Geometry check sheet. Reference: drawing and pictorial views, mm from the part's lowest x, y, z. A direction names the side the tool comes from. Round coordinates to 2 decimals unless told otherwise and drop trailing zeros. Order: outer loops, then holes, each group sorted by start corner. A loop starts at its lowest first (then second) coordinate and runs counter-clockwise, first axis right, second up. Notation, with made-up numbers: (86.5, 24) -> (133.5, 24) arc R16 ccw to (133.5, 41) -> close; hole circle Ø7 at (76, -5). An arc over 180 degrees is marked (long way). Put each result on its own line as item: value.
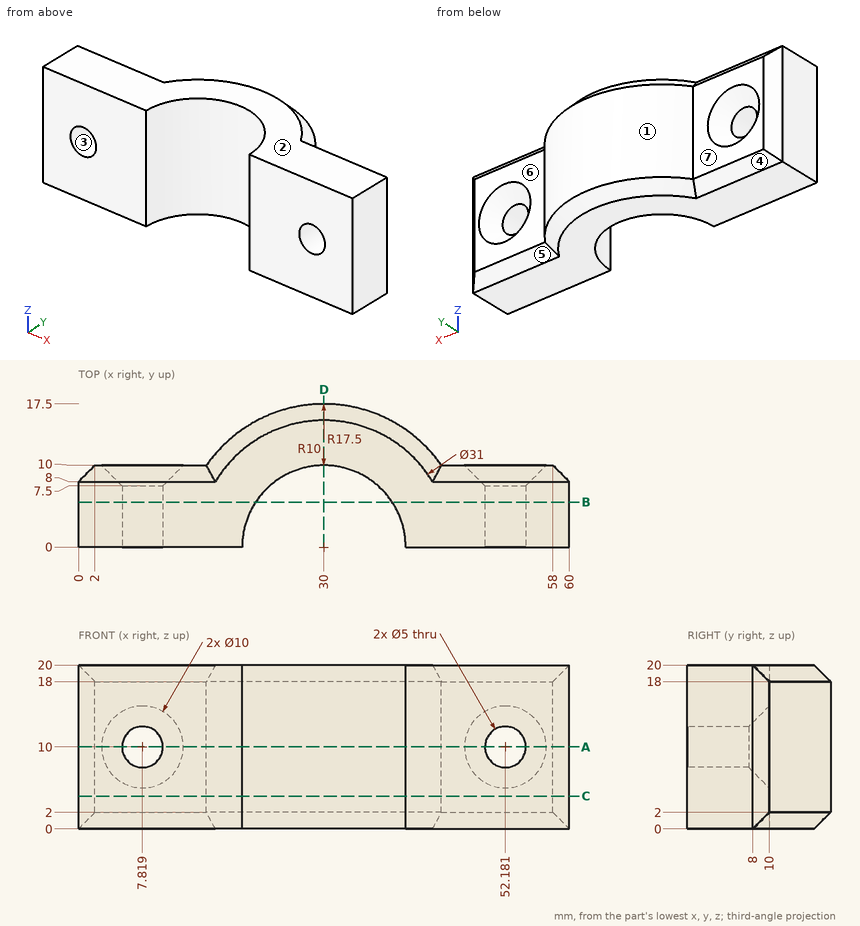
Item 1: Sectioned sample at A-A, the plane z = 10. Record the boundary of the cut face in (x, y).
Geometry check:
outline: (0, 0) -> (5.32, 0) -> (5.32, 7.5) -> (2.82, 10) -> (2, 10) -> (0, 8) -> close; (10.32, 0) -> (20, 0) arc R10 cw to (40, 0) -> (49.68, 0) -> (49.68, 7.5) -> (47.18, 10) -> (44.36, 10) arc R17.5 ccw to (15.64, 10) -> (12.82, 10) -> (10.32, 7.5) -> close; (54.68, 0) -> (60, 0) -> (60, 8) -> (58, 10) -> (57.18, 10) -> (54.68, 7.5) -> close
Item 2: Sectioned sample at B-B, the plane y = 5.5. Record the boundary of the cut face in (x, z), then the cut area to 3 significant figures.
Geometry check:
outline: (0, 0) -> (21.65, 0) -> (21.65, 20) -> (0, 20) -> close; (38.35, 0) -> (60, 0) -> (60, 20) -> (38.35, 20) -> close; hole circle Ø5 at (7.82, 10); hole circle Ø5 at (52.18, 10)
area: 827 mm2
Item 3: Release check for a two-part mould opening along X. For the marked faces 1, 2 and 3 record: pulls with the +X half, pulls with the -X half, needs draft (parallel to the pull), parting line crosses it, or undercut.
Geometry check:
face 1: parting line crosses it
face 2: needs draft
face 3: undercut
Item 4: Sectioned sample at D-D, the plane x = 30. Record the boundary of the cut face in (y, z).
Geometry check:
outline: (10, 0) -> (15.5, 0) -> (17.5, 2) -> (17.5, 18) -> (15.5, 20) -> (10, 20) -> close
Item 5: Material ranges on line 1 along X through (y, z) = (5, 10); line 2 along X through (y, z) = (5.5, 10); line 3 along X through (y, z) = (3.75, 18.5), recorded low to high.
Geometry check:
line 1: 0 to 5.32, 10.32 to 21.34, 38.66 to 49.68, 54.68 to 60
line 2: 0 to 5.32, 10.32 to 21.65, 38.35 to 49.68, 54.68 to 60
line 3: 0 to 20.73, 39.27 to 60
Item 6: Depth check by flat-ended pin: pin 1 Ø11 at (x, z) = (6.5, 6) entering from +Y; pin 2 Ø10 at (x, y) = (9.5, 10) entering from -Z; pin 3 Ø8 at (x, z) = (52.18, 10) entering from +Y. Enter the tip coordinate at first touch or a pass-through.
Geometry check:
pin 1: y = 10
pin 2: z = 0
pin 3: y = 9
Item 7: Sectioned sample at C-C, the plane z = 4. Record the boundary of the cut face in (x, y).
Geometry check:
outline: (0, 0) -> (20, 0) arc R10 cw to (40, 0) -> (60, 0) -> (60, 8) -> (58, 10) -> (44.36, 10) arc R17.5 ccw to (15.64, 10) -> (2, 10) -> (0, 8) -> close
Item 8: Tool access check on the marked faces 4, 5, 6 and 7. Record the directions out of +Z, -Z, +X, -X, +Y, -Y that give a thin tool (end or side, any length) a straight path to the whole face; none if there is none.
Geometry check:
face 4: -Z, -X, +Y
face 5: -Z, +X, +Y
face 6: +Z, -Z, +X, +Y
face 7: +Z, -Z, -X, +Y
